from build123d import *

# Parameters (mm, degrees)
F1_DEPTH     = 40
F2_R         = 5
F2_R_2       = 2.5
F3_DEPTH     = 4
F4_DEPTH     = 15.001
F2_W         = 14
F2_H         = 6
F5_DEPTH     = 10
F2_H_2       = 10
F6_DEPTH     = 10
F7_SIZE      = 9.99999
F8_W         = 10
F8_H         = 10
F8_W_2       = 8
F9_DEPTH     = 15
F10_T4_DEPTH = 61.4336597593


# Not quite as in the source:
# - a fillet or chamfer that OpenCascade refuses, or shapes differently, is made with other operations: its cross-section is extruded or revolved along the edge and cut away or added
# - a fillet or chamfer is up to 0.001 mm smaller than in the source, because OpenCascade refuses the exact size
# - a feature names something its author has since deleted; it is built from what else it names


with BuildPart() as f1:
    # F0 (on Top) → F1 (new body)
    with BuildSketch(Plane.XY):
        Polygon((-20.9070546148, 3.6112386312), (-20.9070546148, 37.6112386312), (-35.9070546148, 37.6112386312), (-35.9070546148, -12.3887613688), (25.0929453852, -12.3887613688), (25.0929453852, 3.6112386312), (17.0929453852, 3.6112386312), (17.0929453852, -2.3887613688), (7.0929453852, -2.3887613688), (7.0929453852, 3.6112386312), (-0.9070546148, 3.6112386312), (-0.9070546148, -2.3887613688), (-10.9070546148, -2.3887613688), (-10.9070546148, 3.6112386312), align=None)
    extrude(amount=F1_DEPTH)

    # F2 (on face) → F3 (cut)
    with BuildSketch(Plane.YZ.offset(-20.9070546148)):
        with Locations((29.6112386312, 9.4117647059)):
            Circle(F2_R)
        with Locations((29.6112386312, 9.4117647059)):
            Circle(F2_R_2, mode=Mode.SUBTRACT)
        with Locations((11.6112386312, 20)):
            Circle(F2_R)
        with Locations((11.6112386312, 20)):
            Circle(F2_R_2, mode=Mode.SUBTRACT)
        with Locations((29.6112386312, 30.5882352941)):
            Circle(F2_R)
        with Locations((29.6112386312, 30.5882352941)):
            Circle(F2_R_2, mode=Mode.SUBTRACT)
    extrude(amount=-F3_DEPTH, mode=Mode.SUBTRACT)

    # F4 (cut, through all): faces of the model
    f4_faces = [f1.faces().sort_by_distance(p)[0] for p in [
        (-20.9070546148, 29.6112386312, 9.4117647059),
        (-20.9070546148, 11.6112386312, 20),
        (-20.9070546148, 29.6112386312, 30.5882352941),
    ]]
    extrude(f4_faces, amount=-F4_DEPTH, mode=Mode.SUBTRACT)

    # F2 (on face) → F5 (join)
    with BuildSketch(Plane.YZ.offset(-20.9070546148)):
        with Locations((10.6112386312, 33)):
            Rectangle(F2_W, F2_H)
    extrude(amount=F5_DEPTH)

    # F2 (on face) → F6 (join)
    with BuildSketch(Plane.YZ.offset(-20.9070546148)):
        with Locations((10.6112386312, 5)):
            Rectangle(F2_W, F2_H_2)
    extrude(amount=F6_DEPTH)

    # F7 (size 10 in the source; OpenCascade refuses exactly that, so slightly less here)
    f7_edges = [f1.edges().sort_by_distance(p)[0] for p in [
        (-10.907055, 17.611239, 33),
    ]]
    chamfer(f7_edges, length=F7_SIZE)

    # F8 (on face) → F9 (join)
    with BuildSketch(Plane(origin=(0, -2.3887613688, 0), x_dir=(-1, 0, 0), z_dir=(0, 1, 0))):
        with Locations((-12.0929453852, 5)):
            Rectangle(F8_W, F8_H)
        with Locations((5.9070546148, 5)):
            Rectangle(F8_W, F8_H)
        with Locations((-3.0929453852, 5)):
            Rectangle(F8_W_2, F8_H)
    extrude(amount=F9_DEPTH)

    # F10: chamfer of 10 on 1 edges, made by hand


with BuildPart() as f10_tool2:
    # F10_s3 → F10_t4 (new body)
    with BuildSketch(Plane.XY.offset(-25.7168298797)):
        Polygon((-20.9070546148, 17.6112386312), (-10.9070546148, 7.6112386312), (-10.9070546148, 17.6112386312), align=None)
    extrude(amount=F10_T4_DEPTH)

    split(bisect_by=Plane.YZ.offset(-20.9070546148), keep=Keep.TOP)

    split(bisect_by=Plane.XZ.offset(-12.6112386312), keep=Keep.BOTTOM)


with BuildPart() as f1_1:
    add(f1.part)

    # F10_t1: cut F10_tool2
    add(f10_tool2.part, mode=Mode.SUBTRACT)


solid = f1_1.part
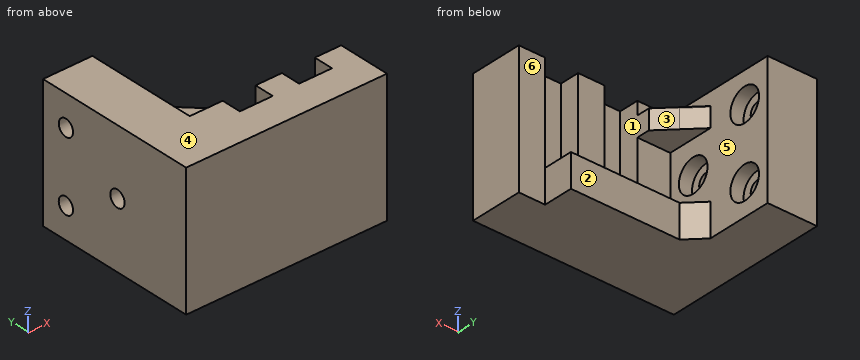
Read the model definition and answer for the solid it produces. Units are mm, in the model's axes. Face numbers are marked on the shaded views. A direction names the side the tool comes from. Give positions to 0.01 mm unless a question says otherwise; leave off trailing zeros. Loops run counter-clockwise (first coordinate to the right, second up) from the corner with the lowest first, then second, coordinate; pieces in that order, holes last. Notation, with made-up numbers: M 81.5,77.25 L 120.5,77.25 A15 ccw 120.5,86.25 Z; hole C 59.25,46.5 d8. An arc over 180 degrees is marked long. Write each question's results on one line, items separated by ' | '.
1. Section B-B on x = 5.5 is taken. Give the vertices of the cut face in (y, z).
Values:
outline: M -12.39,0 L 12.61,0 L 12.61,10 L 3.61,10 L 3.61,40 L -12.39,40 Z
2. Section D-D on y = 20 is taken. Give the vertices of the cut face in (x, z).
Values:
outline: M -35.91,0 L -20.91,0 L -20.91,40 L -35.91,40 Z
3. Given pin 1 (5 mm diameter, centred on x = -14, z = 20.5, fed in from +Y); pin 2 (6.5 mm diameter, centred on y = 29.61, z = 9.41, fed in from -X); pin 3 (1.5 mm diameter, centred on x = 10, z = 19.5, fed in from +Y); pin 4 (3 mm diameter, centred on y = 10.5, z = 22, fed in from +X), each flat-ended and moving along its own axis, determine where each tip first touches the part or whether it passes through.
Values:
pin 1: stops at y = 3.61 | pin 2: stops at x = -35.91 | pin 3: stops at y = -2.39 | pin 4: stops at x = -24.91
4. Straight lines are drawn through the part: line 1 (Z direction, x = -20, y = 4.5); line 2 (X direction, y = 0.5, z = 27); line 3 (Z direction, x = -22, y = 27). For each, find the intervals that lie inside material, in ascending order. Write a range as [from, to].
Values:
line 1: z = [0, 10], [30, 36] | line 2: x = [-35.91, -10.91], [-0.91, 7.09], [17.09, 25.09] | line 3: z = [0, 5.15], [13.68, 26.32], [34.85, 40]
5. Section A-A on z = 20 is taken. Give the vertices of the cut face in (x, y).
Values:
outline: M -35.91,-12.39 L 25.09,-12.39 L 25.09,3.61 L 17.09,3.61 L 17.09,-2.39 L 7.09,-2.39 L 7.09,3.61 L -0.91,3.61 L -0.91,-2.39 L -10.91,-2.39 L -10.91,3.61 L -20.91,3.61 L -20.91,6.61 L -24.91,6.61 L -24.91,9.11 L -35.91,9.11 Z; M -35.91,14.11 L -24.91,14.11 L -24.91,16.61 L -20.91,16.61 L -20.91,37.61 L -35.91,37.61 Z
6. The mould has two halves that part along Z. Classify the marked faces 4, 5 and 6: pulls with the +Z half, pulls with the -Z half, needs draft (parallel to the pull), parting line crosses it, or undercut.
Values:
face 4: pulls with the +Z half | face 5: undercut | face 6: needs draft
7. A tool of negligible diameter and unlimited length cuts with its end or side. For the marked faces 1, 2 and 3, from which of +Z, -Z, +X, -X, +Y, -Y can it reach the whole face along a straight path? Write none if from no direction.
Values:
face 1: +Z, +Y | face 2: +Z, -Z, +X, +Y | face 3: +Z, +X, +Y
